CAD build for the part. Positions are in the model's coordinates, mm. A direction names the side the tool comes from. Coordinates: 2 decimals unless noted, no trailing zeros. Write each loop counter-clockwise with the first axis right and the second up, starting at its lowest first coordinate (ties: lowest second). Pieces come first, ordered by that corner, then holes. Notation, with made-up numbers: (56.25, 64) - (100.25, 64) arc R14 cw to (100.25, 84) - close; hole circle Ø9 at (-25.75, 54). An arc over 180 degrees is marked (long way). One line per question, with ' | ' between items. Start each with the question number.
1. Which spindle directions (+Z, -Z, +X, -X, +Y, -Y) get a long thin tool onto all of the face, cutting with end or side? Do faces 4 (the cylindrical face through (0.007, -6.096, -4.268)), 5 (the cylindrical face through (1.72, -5.85, -4.27)), 6 (the cylindrical face through (1.71, 5.85, -4.27)), 7 (the flat face through (-6, -2, -7.874)). Say none if no direction does.
2. Flat gauge pins, fed straight in: P1, Ø2, axis at y = -7, z = -6.5, coming from the +X side; P2, Ø2, axis at y = 1.5, z = -2, coming from the +X side; P3, Ø1, axis at x = -1.5, z = -2.5, coming from the +Y side. Where does each tip first touch, or does it go through?
3. Band-saw the part on C-C, the plane z = -10.25. Write the cut outline in (x, y) (3 decimals).
4. Probe line 1 (Y direction, x = 0, z = -9) (3 decimals); line 2 (Z direction, x = -5, y = -6.25); line 3 (Y direction, x = -1.5, z = -4). List the from-to ranges inside material, lowest first.
5. Band-saw the part on D-D, the plane y = 6.75. Write the cut outline in (x, z), then the cut area to 3 significant figures.
6. Two-plate mould, pull along X, no slides. Class faces 1 (the cylindrical face through (-6.035, 0.861, -4.268)), 2 (the cylindrical face through (3.302, -5.125, -4.268)), 3 (the cylindrical face through (-0.69, -3.1, -6.51)): +X half, -X half, draft (parallel to the pull), parting line (faces both ways), or undercut.
7. Band-saw the part on A-A, the plane y = 0. Write the cut outline in (x, z) (3 decimals), then the cut area to 3 significant figures.
8. Band-saw the part on B-B, the plane x = 0. Write the cut outline in (y, z) (3 decimals), then the cut area to 3 significant figures.
from build123d import *

# Parameters (mm, degrees)
SKETCH1_R           = 8.636
BOSS_EXTRUDE1_DEPTH = 0.762
SKETCH2_R           = 6.096
BOSS_EXTRUDE2_DEPTH = 7.112
SKETCH3_R           = 8.636
BOSS_EXTRUDE3_DEPTH = 5.334
SKETCH4_R           = 3.175
CUT_EXTRUDE1_DEPTH  = 25.654
SKETCH5_W           = 7.112
SKETCH5_H           = 0.762
CUT_EXTRUDE2_DEPTH  = 0.254
CIRPATTERN1_COUNT   = 22


with BuildPart() as part:
    # Sketch1 → Boss-Extrude1 (new body)
    with BuildSketch(Plane.XY):
        Circle(SKETCH1_R)
    extrude(amount=-BOSS_EXTRUDE1_DEPTH)

    # Sketch2 → Boss-Extrude2 (add)
    with BuildSketch(Plane(origin=(0, 0, -0.762), x_dir=(-1, 0, 0), z_dir=(0, 0, -1))):
        Circle(SKETCH2_R)
    extrude(amount=BOSS_EXTRUDE2_DEPTH)

    # Sketch3 → Boss-Extrude3 (add)
    with BuildSketch(Plane(origin=(0, 0, -7.874), x_dir=(-1, 0, 0), z_dir=(0, 0, -1))):
        Circle(SKETCH3_R)
    extrude(amount=BOSS_EXTRUDE3_DEPTH)

    # Sketch4 → Cut-Extrude1 (cut)
    with BuildSketch(Plane.XY):
        Circle(SKETCH4_R)
    extrude(amount=-CUT_EXTRUDE1_DEPTH, mode=Mode.SUBTRACT)

    # Sketch5 → Cut-Extrude2 (cut)
    with BuildSketch(Plane.ZY.offset(6.096)):
        with Locations((-4.318, 0)):
            Rectangle(SKETCH5_W, SKETCH5_H)
    cut_extrude2 = extrude(amount=-CUT_EXTRUDE2_DEPTH, mode=Mode.SUBTRACT)

    # CirPattern1: Cut-Extrude2 ×22 about axis
    cirpattern1_axis = Axis((0, 0, 0), (0, 0, 1))
    for i in range(1, CIRPATTERN1_COUNT):
        add(cut_extrude2.rotate(cirpattern1_axis, i * 360 / CIRPATTERN1_COUNT), mode=Mode.SUBTRACT)


solid = part.part
Filled in:
1) face 4: -Y | face 5: +X, -Y | face 6: +X, +Y | face 7: none
2) P1: stops at x = 0.49 | P2: stops at x = 6.08 | P3: stops at y = 5.97
3) outline: circle Ø17.272 at (0, 0); hole circle Ø6.35 at (0, 0)
4) line 1: y = -8.636 to -3.175, 3.175 to 8.636 | line 2: z = -13.21 to -7.87, -0.76 to 0 | line 3: y = -5.91 to -2.8, 2.8 to 5.91
5) outline: (-5.39, -13.21) - (5.39, -13.21) - (5.39, -7.87) - (-5.39, -7.87) - close; (-5.39, -0.76) - (5.39, -0.76) - (5.39, 0) - (-5.39, 0) - close | area: 65.7 mm²
6) face 1: -X half | face 2: +X half | face 3: undercut
7) outline: (-8.636, -13.208) - (-3.175, -13.208) - (-3.175, 0) - (-8.636, 0) - (-8.636, -0.762) - (-5.842, -0.762) - (-5.842, -7.874) - (-8.636, -7.874) - close; (3.175, -13.208) - (8.636, -13.208) - (8.636, -7.874) - (5.842, -7.874) - (5.842, -0.762) - (8.636, -0.762) - (8.636, 0) - (3.175, 0) - close | area: 105 mm²
8) outline: (-8.636, -13.208) - (-3.175, -13.208) - (-3.175, 0) - (-8.636, 0) - (-8.636, -0.762) - (-6.096, -0.762) - (-6.096, -7.874) - (-8.636, -7.874) - close; (3.175, -13.208) - (8.636, -13.208) - (8.636, -7.874) - (6.096, -7.874) - (6.096, -0.762) - (8.636, -0.762) - (8.636, 0) - (3.175, 0) - close | area: 108 mm²
